Here's the drawing with two shaded views (mm, measured from the low corner). I have some questions. A direction names the side the tool comes from. Coordinates: 2 decimals unless noted, no trailing zeros. Write each loop counter-clockwise with the first axis right and the second up, starting at its lowest first coordinate (ties: lowest second). Pieces come first, ordered by that corner, then holes.
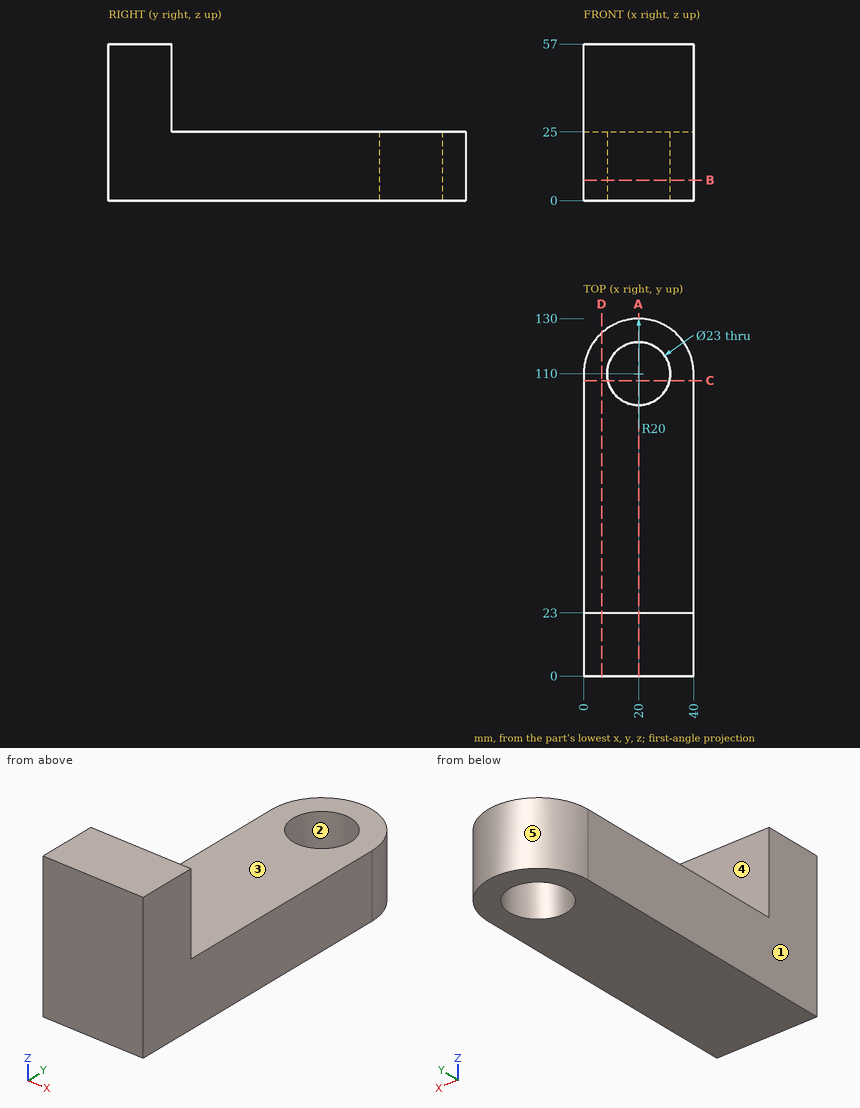
1. For pin 1 (10 mm diameter, centred on x = 17, y = 48.5, fed in from +Z); pin 2 (5 mm diameter, centred on x = 19, z = 38.5, fed in from +Y); pin 3 (12 mm diameter, centred on y = 80, z = 25.5, fed in from +X), each with a flat end and sliding along its axis, tell me the tip position at first contact or that it passes through.
Verdict:
pin 1: stops at z = 25
pin 2: stops at y = 23
pin 3: stops at x = 40
2. If we mould it in two halves opening along X, with no side actions, what happens to the marked faces 1, 2 and 3? For each: pulls with the +X half, pulls with the -X half, needs draft (parallel to the pull), parting line crosses it, or undercut.
Verdict:
face 1: pulls with the -X half
face 2: undercut
face 3: needs draft
3. On a 3-axis mill with a long thin cutter (end or side, diameter ignored), from which of +Z, -Z, +X, -X, +Y, -Y can I reach the whole of each face in a straight line? I mean the marked faces 4 and 5. Say none if no direction works.
Verdict:
face 4: +Z, +X, -X, +Y
face 5: +Z, -Z, +Y
4. I want a section at D-D on x = 6.5. Please give me the cut outline in (y, z).
Verdict:
outline: (0, 0) - (124.76, 0) - (124.76, 25) - (23, 25) - (23, 57) - (0, 57) - close
5. I want a section at A-A on x = 20. Please give me the cut outline in (y, z), plus the area to 3 significant figures.
Verdict:
outline: (0, 0) - (98.5, 0) - (98.5, 25) - (23, 25) - (23, 57) - (0, 57) - close; (121.5, 0) - (130, 0) - (130, 25) - (121.5, 25) - close
area: 3,410 mm2
6. I want a section at C-C on y = 107.5. Please give me the cut outline in (x, z), plus the area to 3 significant figures.
Verdict:
outline: (0, 0) - (8.78, 0) - (8.78, 25) - (0, 25) - close; (31.22, 0) - (40, 0) - (40, 25) - (31.22, 25) - close
area: 439 mm2
7. I want a section at B-B on z = 7.5. Please give me the cut outline in (x, y), plus the area to 3 significant figures.
Verdict:
outline: (0, 0) - (40, 0) - (40, 110) arc R20 ccw to (0, 110) - close; hole circle Ø23 at (20, 110)
area: 4,610 mm2
8. Please list where these lines run through material, in increasing order: line 1 along X through (y, z) = (110, 17); line 2 along Y through (x, z) = (20, 6); line 3 along Z through (x, y) = (29, 124.5).
Verdict:
line 1: x = 0 to 8.5, 31.5 to 40
line 2: y = 0 to 98.5, 121.5 to 130
line 3: z = 0 to 25
